Part model, mm, in its own coordinate system. A direction names the side the tool comes from. Coordinates: 2 decimals unless noted, no trailing zeros. Loops run counter-clockwise (first coordinate to the right, second up) from the corner with the lowest first, then second, coordinate; pieces in that order, holes last. Notation, with made-up numbers: (48, 21.25) -> (65, 21.25) arc R17 ccw to (65, 34.25) -> close; hole circle Ø3 at (29, 64). An arc over 180 degrees is marked (long way). Use one line per item in the form item = value. Start each with the question number.
(1) 3-axis set-ups, long thin cutter, end or side, ignore diameter. For faces 4 (the cylindrical face through (2.06, -7.89, -29.5)), 5 (the cylindrical face through (6.07, -14.88, 3.3)): which of +Z, -Z, +X, -X, +Y, -Y reach the whole face in a straight line?
(2) Band-saw the part on D-D on z = -122.5. Give the cut face in (x, y).
(3) Band-saw the part on B-B on x = 1.25. Give the cut face in (y, z), then the cut area to 3 significant figures.
(4) Band-saw the part on C-C on y = 0. Count the separate pieces of the cut face and the enclosed holes in it, then the cut area to 3 significant figures.
(5) Band-saw the part on A-A on z = -76.2. Give the cut face in (x, y), then the cut area to 3 significant figures.
(6) Drill centre lines: L1, parallel to Y at x = 2.55, z = -101.6; L2, parallel to X at y = 11, z = -36; L3, parallel to Z at x = 4.5, y = -8. Where is each one in solid material? Low to high. Write a range as [from, to].
(7) Mould opens along Y. For faces 1 (the cylindrical face through (2.004, -0.447, 20.315)), 2 (the cylindrical face through (2.06, 0.39, -118.12)), 3 (the flat face through (2, 20.32, -88)) say: +Y half, -Y half, draft (parallel to the pull), parting line (faces both ways), or undercut.
(8) Pin check, flat tips, straight feed: P1, Ø3, axis at y = 14, z = -97.5, coming from the +X side; P2, Ø2, axis at y = -5, z = -171.5, coming from the -X side; P3, Ø1.5, axis at x = 5.5, y = -13.5, coming from the -Z side. Stop position of each tip, or through.
```python
from build123d import *

# Parameters (mm, degrees)
BOSS_EXTRUDE1_DEPTH = 4.064
SKETCH2_R           = 15.24
BOSS_EXTRUDE2_DEPTH = 4.064
SKETCH3_R           = 8.89
CUT_EXTRUDE1_DEPTH  = 5.064
LPATTERN1_COUNT     = 6
LPATTERN1_PITCH     = 25.4


with BuildPart() as part:
    # Sketch1 → Boss-Extrude1 (new body)
    with BuildSketch(Plane(origin=(0, 0, 0), x_dir=(0, 0, -1), z_dir=(1, 0, 0))):
        with BuildLine():
            Line((0, 20.32), (177.8, 20.32))
            ThreePointArc((177.8, 20.32), (198.12, 0), (177.8, -20.32))
            Line((177.8, -20.32), (0, -20.32))
            ThreePointArc((0, -20.32), (-20.32, 0), (0, 20.32))
        make_face()
    extrude(amount=BOSS_EXTRUDE1_DEPTH)

    # Sketch2 → Boss-Extrude2 (add)
    with BuildSketch(Plane(origin=(4.064, 0, 0), x_dir=(0, 0, -1), z_dir=(1, 0, 0))):
        Circle(SKETCH2_R)
        with Locations((177.8, 0)):
            Circle(SKETCH2_R)
    extrude(amount=BOSS_EXTRUDE2_DEPTH)

    # Sketch3 → Cut-Extrude1 (cut, through all)
    with BuildSketch(Plane(origin=(4.064, 0, 0), x_dir=(0, 0, -1), z_dir=(1, 0, 0))):
        with Locations((25.4, 0)):
            Circle(SKETCH3_R)
    cut_extrude1 = extrude(amount=-CUT_EXTRUDE1_DEPTH, mode=Mode.SUBTRACT)

    # LPattern1: Cut-Extrude1 ×6
    with Locations(*[(0, 0, -i * LPATTERN1_PITCH) for i in range(1, LPATTERN1_COUNT)]):
        add(cut_extrude1, mode=Mode.SUBTRACT)


solid = part.part
```
A:
q1.face_4 = +X, -X
q1.face_5 = +X
q2.outline = (0, -20.32) -> (4.06, -20.32) -> (4.06, -7.67) -> (0, -7.67) -> close; (0, 7.67) -> (4.06, 7.67) -> (4.06, 20.32) -> (0, 20.32) -> close
q3.outline = (-20.32, -177.8) arc R20.32 ccw to (20.32, -177.8) -> (20.32, 0) arc R20.32 ccw to (-20.32, 0) -> close; hole circle Ø17.78 at (0, -152.4); hole circle Ø17.78 at (0, -127); hole circle Ø17.78 at (0, -101.6); hole circle Ø17.78 at (0, -76.2); hole circle Ø17.78 at (0, -50.8); hole circle Ø17.78 at (0, -25.4)
q3.area = 7,030 mm²
q4.separate_pieces = 7
q4.enclosed_holes = 0
q4.area = 702 mm²
q5.outline = (0, -20.32) -> (4.06, -20.32) -> (4.06, -8.89) -> (0, -8.89) -> close; (0, 8.89) -> (4.06, 8.89) -> (4.06, 20.32) -> (0, 20.32) -> close
q5.area = 92.9 mm²
q6.L1 = [-20.32, -8.89], [8.89, 20.32]
q6.L2 = [0, 4.06]
q6.L3 = [-190.77, -164.83], [-12.97, 12.97]
q7.face_1 = parting line
q7.face_2 = undercut
q7.face_3 = +Y half
q8.P1 = 4.06
q8.P2 = 0
q8.P3 = -186.15
